from build123d import *

# Parameters (mm, degrees)
F1_DEPTH = 82.55
F2_R     = 9.7282
F3_DEPTH = 38.101


with BuildPart() as f1:
    # F0 (on Front) → F1 (new body, symmetric)
    with BuildSketch(Plane.XZ):
        with BuildLine():
            ThreePointArc((19.05, 13.6652), (17.472829, 17.472829), (13.6652, 19.05))
            Line((13.6652, 19.05), (-13.6652, 19.05))
            ThreePointArc((-13.6652, 19.05), (-17.472829, 17.472829), (-19.05, 13.6652))
            Line((-19.05, 13.6652), (-19.05, -13.6652))
            ThreePointArc((-19.05, -13.6652), (-17.472829, -17.472829), (-13.6652, -19.05))
            Line((-13.6652, -19.05), (13.6652, -19.05))
            ThreePointArc((13.6652, -19.05), (17.472829, -17.472829), (19.05, -13.6652))
            Line((19.05, -13.6652), (19.05, 13.6652))
        make_face()
        with BuildLine():
            Line((-13.6652, 16.002), (13.6652, 16.002))
            ThreePointArc((13.6652, 16.002), (15.317567, 15.317567), (16.002, 13.6652))
            Line((16.002, 13.6652), (16.002, -13.6652))
            ThreePointArc((16.002, -13.6652), (15.317567, -15.317567), (13.6652, -16.002))
            Line((13.6652, -16.002), (-13.6652, -16.002))
            ThreePointArc((-13.6652, -16.002), (-15.317567, -15.317567), (-16.002, -13.6652))
            Line((-16.002, -13.6652), (-16.002, 13.6652))
            ThreePointArc((-16.002, 13.6652), (-15.317567, 15.317567), (-13.6652, 16.002))
        make_face(mode=Mode.SUBTRACT)
    extrude(amount=F1_DEPTH, both=True)

    # F2 (on face) → F3 (cut, through all)
    with BuildSketch(Plane(origin=(-19.05, 0, 0), x_dir=(0, -1, 0), z_dir=(-1, 0, 0))):
        Circle(F2_R)
    extrude(amount=-F3_DEPTH, mode=Mode.SUBTRACT)


solid = f1.part
The model under review builds one solid part; all positions refer to its coordinate system, in mm. A direction names the side the tool comes from. Round coordinates to 2 decimals unless told otherwise and drop trailing zeros. Loops run counter-clockwise (first coordinate to the right, second up) from the corner with the lowest first, then second, coordinate; pieces in that order, holes last. Notation, with made-up numbers: M -39.5,68 L 7.5,68 A21 cw 7.5,83 Z; hole C 63,59 d9. An arc over 180 degrees is marked long. Answer as CSV lines item,"result".
1. Draft analysis for pull direction X (two halves, no side actions). For faces 1 (the face through (0, -1, -19.05)), 2 (the face through (19.05, -1, 12)), 3 (the face through (0, -1, 16.002)), 4 (the face through (16.002, -1, -12)), state which applies: pulls with the +X half, pulls with the -X half, needs draft (parallel to the pull), parting line crosses it, or undercut.
Outcome:
face 1,"needs draft"
face 2,"pulls with the +X half"
face 3,"undercut"
face 4,"undercut"
2. We need section B-B (x = 5). Give the boundary of the cut face in (y, z), plus the area to 3 significant figures.
Outcome:
outline,"M -82.55,-19.05 L 82.55,-19.05 L 82.55,-16 L -82.55,-16 Z; M -82.55,16 L 82.55,16 L 82.55,19.05 L -82.55,19.05 Z"
area,"1,010 mm2"
3. To check wall thickness, follow L1, parallel to Z at x = -13, y = -67; L2, parallel to Z at x = -18, y = 0. State the ranges of each line that lie inside material, in increasing order. Write a range as [from, to].
Outcome:
L1,"z = [-19.05, -16], [16, 19.05]"
L2,"z = [-16.86, -9.73], [9.73, 16.86]"
4. We need section D-D (y = 49). Give the boundary of the cut face in (x, z), plus the area to 3 significant figures.
Outcome:
outline,"M -19.05,-13.67 A5.38 ccw -13.67,-19.05 L 13.67,-19.05 A5.38 ccw 19.05,-13.67 L 19.05,13.67 A5.38 ccw 13.67,19.05 L -13.67,19.05 A5.38 ccw -19.05,13.67 Z; hole M -16,-13.67 A2.34 ccw -13.67,-16 L 13.67,-16 A2.34 ccw 16,-13.67 L 16,13.67 A2.34 ccw 13.67,16 L -13.67,16 A2.34 ccw -16,13.67 Z"
area,"407 mm2"
5. We need section A-A (z = 0). Give the boundary of the cut face in (x, y), plus the area to 3 significant figures.
Outcome:
outline,"M -19.05,-82.55 L -16,-82.55 L -16,-9.73 L -19.05,-9.73 Z; M -19.05,9.73 L -16,9.73 L -16,82.55 L -19.05,82.55 Z; M 16,-82.55 L 19.05,-82.55 L 19.05,-9.73 L 16,-9.73 Z; M 16,9.73 L 19.05,9.73 L 19.05,82.55 L 16,82.55 Z"
area,"888 mm2"
6. Insertion check: pin 1 Ø15.5 at (y, z) = (0, 0) entering from +X. The pin has a flat end and moves straight along its axis. Give the tip position at first contact, or say it passes through.
Outcome:
pin 1,"passes through"
7. We need section C-C (y = 0). Give the boundary of the cut face in (x, z).
Outcome:
outline,"M -19.05,-13.67 A5.38 ccw -13.67,-19.05 L 13.67,-19.05 A5.38 ccw 19.05,-13.67 L 19.05,-9.73 L 16,-9.73 L 16,-13.67 A2.34 cw 13.67,-16 L -13.67,-16 A2.34 cw -16,-13.67 L -16,-9.73 L -19.05,-9.73 Z; M -19.05,9.73 L -16,9.73 L -16,13.67 A2.34 cw -13.67,16 L 13.67,16 A2.34 cw 16,13.67 L 16,9.73 L 19.05,9.73 L 19.05,13.67 A5.38 ccw 13.67,19.05 L -13.67,19.05 A5.38 ccw -19.05,13.67 Z"
8. For faces 5 (the face through (-19.05, -1, -12)), 6 (the face through (0, -1, -16.002)), list the 3-axis set-ups (+Z, -Z, +X, -X, +Y, -Y) from which the entire face can be reached by the end or side of a thin tool; tool diameter is ignored.
Outcome:
face 5,"+Z, -Z, -X, +Y, -Y"
face 6,"+Y, -Y"
